Input: part model. Units: mm. Frame: model coordinates. Face numbers are marked on the shaded views. A direction names the side the tool comes from. Coordinates: 2 decimals unless noted, no trailing zeros. Answer as CSV lines item,"result".
from build123d import *

# Parameters (mm, degrees)
CUT_EXTRUDE1_START           = -3.6
CUT_EXTRUDE1_DEPTH           = 3.6
CUT_EXTRUDE2_DEPTH           = 3.6
M3_CLEARANCE_HOLE3_D         = 3.4
CHAMFER2_SIZE                = 1
M4_CLEARANCE_HOLE2_D         = 4.3
CIRPATTERN2_COUNT            = 6
CHAMFER2_OF_CIRPATTERN2_SIZE = 1
FILLET1_R                    = 0.4
CHAMFER1_SIZE                = 0.4


with BuildPart() as part:
    # Sketch8 → Revolve1 (revolve)
    with BuildSketch(Plane.XY, mode=Mode.PRIVATE) as revolve1_sk:
        Polygon((8.1, 0), (8.1, 4.8), (7.7, 5.2), (7.7, 6), (17.6, 6), (17.6, 0), align=None)
    revolve(revolve1_sk.sketch.rotate(Axis((0, 16.972685485, 0), (0, -1, 0)), 180), axis=Axis((0, 16.972685485, 0), (0, -1, 0)))

    # Sketch2 → Cut-Extrude1 (cut)
    with BuildSketch(Plane(origin=(0, 6, 0), x_dir=(1, 0, 0), z_dir=(0, 1, 0)).offset(CUT_EXTRUDE1_START)):
        with BuildLine():
            Line((13.5, 3.7), (17.206684748, 3.7))
            ThreePointArc((17.206684748, 3.7), (17.6, 0), (17.206684748, -3.7))
            Line((17.206684748, -3.7), (13.5, -3.7))
            ThreePointArc((13.5, -3.7), (9.8, 0), (13.5, 3.7))
        make_face()
    cut_extrude1 = extrude(amount=CUT_EXTRUDE1_DEPTH, mode=Mode.SUBTRACT)

    # Sketch5 → Cut-Extrude2 (cut)
    with BuildSketch(Plane.XZ):
        Polygon((2.8, -14.616580754), (2.8, -11.383419246), (0, -9.766838493), (-2.8, -11.383419246), (-2.8, -14.616580754), (0, -16.233161507), align=None)
    cut_extrude2 = extrude(amount=-CUT_EXTRUDE2_DEPTH, mode=Mode.SUBTRACT)

    # M3 Clearance Hole3 (through all)
    with Locations(Plane(origin=(0, 6, 0), x_dir=(1, 0, 0), z_dir=(0, 1, 0))):
        with Locations((0, 13)):
            m3_clearance_hole3 = Hole(M3_CLEARANCE_HOLE3_D / 2)

    # Chamfer2
    chamfer2_edges = [part.edges().sort_by_distance(p)[0] for p in [
        (1.7, 3.6, -13),
    ]]
    chamfer(chamfer2_edges, length=CHAMFER2_SIZE)

    # M4 Clearance Hole2 (through all)
    with Locations(Plane(origin=(0, 2.4, 0), x_dir=(1, 0, 0), z_dir=(0, 1, 0))):
        with Locations((13.5, 0)):
            m4_clearance_hole2 = Hole(M4_CLEARANCE_HOLE2_D / 2)

    # CirPattern2: Cut-Extrude1, Cut-Extrude2, M3 Clearance Hole3, M4 Clearance Hole2 ×6 about axis
    cirpattern2_axis = Axis((0, 0, 0), (0, 1, 0))
    add([cut_extrude1.rotate(cirpattern2_axis, i * 360 / CIRPATTERN2_COUNT) for i in range(1, CIRPATTERN2_COUNT)], mode=Mode.SUBTRACT)
    add([cut_extrude2.rotate(cirpattern2_axis, i * 360 / CIRPATTERN2_COUNT) for i in range(1, CIRPATTERN2_COUNT)], mode=Mode.SUBTRACT)
    add([m3_clearance_hole3.rotate(cirpattern2_axis, i * 360 / CIRPATTERN2_COUNT) for i in range(1, CIRPATTERN2_COUNT)], mode=Mode.SUBTRACT)
    add([m4_clearance_hole2.rotate(cirpattern2_axis, i * 360 / CIRPATTERN2_COUNT) for i in range(1, CIRPATTERN2_COUNT)], mode=Mode.SUBTRACT)

    # Chamfer2 of CirPattern2
    chamfer2_of_cirpattern2_edges = [part.edges().sort_by_distance(p)[0] for p in [
        (-10.408330249, 3.6, -7.972243186),
        (-12.108330249, 3.6, 5.027756814),
        (-1.7, 3.6, 13),
        (10.408330249, 3.6, 7.972243186),
        (12.108330249, 3.6, -5.027756814),
    ]]
    chamfer(chamfer2_of_cirpattern2_edges, length=CHAMFER2_OF_CIRPATTERN2_SIZE)

    # Fillet1
    fillet1_edges = [part.edges().sort_by_distance(p)[0] for p in [
        (-5.39904838, 4.2, 16.751426106),
        (-11.807636368, 4.2, 13.051426106),
        (11.807636368, 4.2, 13.051426106),
        (5.39904838, 4.2, 16.751426106),
        (17.206684748, 4.2, -3.7),
        (17.206684748, 4.2, 3.7),
        (5.39904838, 4.2, -16.751426106),
        (11.807636368, 4.2, -13.051426106),
        (-11.807636368, 4.2, -13.051426106),
        (-5.39904838, 4.2, -16.751426106),
        (-17.206684748, 4.2, 3.7),
        (-17.206684748, 4.2, -3.7),
    ]]
    fillet(fillet1_edges, radius=FILLET1_R)

    # Chamfer1
    chamfer1_edges = [part.edges().sort_by_distance(p)[0] for p in [
        (-4.9, 6, 8.487048957),
        (-10.755341767, 6, 11.228798393),
        (4.9, 6, 8.487048957),
        (4.346753779, 6, 14.928798393),
        (9.8, 6, 0),
        (15.102095545, 6, 3.7),
        (-4.346753779, 6, 14.928798393),
        (4.346753779, 6, -14.928798393),
        (0, 6, -17.6),
        (-10.755341767, 6, -11.228798393),
        (-15.242047107, 6, -8.8),
        (-15.102095545, 6, 3.7),
        (-15.242047107, 6, 8.8),
        (0, 6, 17.6),
        (10.755341767, 6, 11.228798393),
        (15.242047107, 6, 8.8),
        (15.102095545, 6, -3.7),
        (15.242047107, 6, -8.8),
        (5.172538285, 6, 16.665418113),
        (11.846406308, 6, 12.812258614),
        (17.018944594, 6, 3.8531595),
        (17.018944594, 6, -3.8531595),
        (11.846406308, 6, -12.812258614),
        (5.172538285, 6, -16.665418113),
        (-5.172538285, 6, -16.665418113),
        (-11.846406308, 6, -12.812258614),
        (-17.018944594, 6, -3.8531595),
        (-17.018944594, 6, 3.8531595),
        (-11.846406308, 6, 12.812258614),
        (-5.172538285, 6, 16.665418113),
        (4.9, 6, -8.487048957),
        (10.755341767, 6, -11.228798393),
        (-4.9, 6, -8.487048957),
        (-4.346753779, 6, -14.928798393),
        (-9.8, 6, 0),
        (-15.102095545, 6, -3.7),
    ]]
    chamfer(chamfer1_edges, length=CHAMFER1_SIZE - 0.0001)  # a hair under: the kernel refuses the full size


solid = part.part
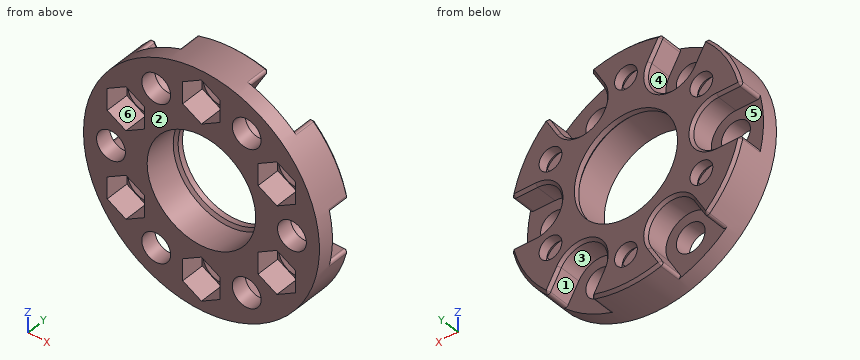
1. Mould query, pull axis Z, two halves, no side actions, for the marked faces 1, 2 and 3. Classes: released by +Z, released by -Z, zero draft, split by the parting line, or undercut.
Findings:
face 1,"released by -Z"
face 2,"zero draft"
face 3,"undercut"
2. Contact query for flat-ended pins moving along their axis: pin 1 (1.5 mm diameter, centred on x = 2, y = 3.5, fed in from -Z); pin 2 (2 mm diameter, centred on x = -11.26, z = -6.5, fed in from +Y); pin 3 (5.5 mm diameter, centred on x = 0, z = -13, fed in from -Y); pin 4 (1.6 mm diameter, centred on x = 14.5, y = 4, fed in from +Z). Output: stop coordinate, or through.
Findings:
pin 1,"stops at z = -17.56"
pin 2,"passes through"
pin 3,"stops at y = 3.6"
pin 4,"stops at z = 11.05"
3. Reachability of the marked faces 4, 5 and 6 from +Z, -Z, +X, -X, +Y, -Y: full face, straight path, thin tool, end or side. Return the list, or none.
Findings:
face 4,"+Y"
face 5,"-X, +Y"
face 6,"-Y"
4. Cut plane A-A (z = 0.5). State how many separate pieces and enclosed holes the cut face has, plus the area to 3 significant figures.
Findings:
separate pieces,"4"
enclosed holes,"0"
area,"38.8 mm2"
5. Ray query, line 1 along Z through (x, y) = (0, 5.45); line 2 along X through (y, z) = (3.75, 8.5); line 3 along Z through (x, y) = (0, 2). Return the intervals inside material, ascending.
Findings:
line 1,"z = -17.6 to -14.7, -11.3 to -7.7, 7.7 to 11.3, 14.7 to 17.6"
line 2,"x = -15.41 to -12.84, -9.68 to -8.62, -4.88 to 4.88, 8.62 to 9.68, 12.84 to 15.41"
line 3,"z = -17.6 to -16.23, -9.77 to -8.1, 8.1 to 9.77, 16.23 to 17.6"
